Geometry check sheet. Reference: the model listing, model coordinates, mm. Face numbers are marked on the shaded views. A direction names the side the tool comes from. Give positions to 0.01 mm unless a question says otherwise; leave off trailing zeros. Loops run counter-clockwise (first coordinate to the right, second up) from the corner with the lowest first, then second, coordinate; pieces in that order, holes last.
```python
from build123d import *

# Parameters (mm, degrees)
F0_W        = 42
F0_H        = 42
F0_R        = 1.4
F0_R_2      = 11.5
F1_DEPTH    = 5
F2_T        = 2.5
F3_T1_DEPTH = 5
F4_DEPTH    = 5
F5_DEPTH    = 25


# Not quite as in the source:
# - a fillet or chamfer that OpenCascade refuses, or shapes differently, is made with other operations: its cross-section is extruded or revolved along the edge and cut away or added


with BuildPart() as f1:
    # F0 (on Top) → F1 (new body)
    with BuildSketch(Plane.XY):
        with Locations((-20.8238260887, 8.1392613277)):
            Rectangle(F0_W, F0_H)
        with Locations((-36.3238260887, -7.3607386723)):
            Circle(F0_R, mode=Mode.SUBTRACT)
        with Locations((-5.3238260887, -7.3607386723)):
            Circle(F0_R, mode=Mode.SUBTRACT)
        with Locations((-36.3238260887, 23.6392613277)):
            Circle(F0_R, mode=Mode.SUBTRACT)
        with Locations((-20.8238260887, 8.1392613277)):
            Circle(F0_R_2, mode=Mode.SUBTRACT)
        with Locations((-5.3238260887, 23.6392613277)):
            Circle(F0_R, mode=Mode.SUBTRACT)
        with Locations((-20.8238260887, 8.1392613277)):
            Circle(F0_R_2)
        with Locations((-36.3238260887, 23.6392613277)):
            Circle(F0_R)
        with Locations((-5.3238260887, 23.6392613277)):
            Circle(F0_R)
        with Locations((-5.3238260887, -7.3607386723)):
            Circle(F0_R)
        with Locations((-36.3238260887, -7.3607386723)):
            Circle(F0_R)
    extrude(amount=F1_DEPTH)

    # F2
    f2_openings = [f1.faces().sort_by_distance(p)[0] for p in [
        (-20.823826, 8.139261, 5),
    ]]
    offset(amount=F2_T, openings=f2_openings, kind=Kind.INTERSECTION)

    # F3: chamfer of 5 on 4 edges, made by hand

    # F3_s2 → F3_t1 (join)
    with BuildSketch(Plane.XY):
        Polygon((0.1761739113, -7.8607386723), (-4.8238260887, -12.8607386723), (0.1761739113, -12.8607386723), align=None)
        Polygon((0.1761739113, 24.1392613277), (-4.8238260887, 29.1392613277), (0.1761739113, 29.1392613277), align=None)
        Polygon((-36.8238260887, 29.1392613277), (-41.8238260887, 24.1392613277), (-41.8238260887, 29.1392613277), align=None)
        Polygon((-41.8238260887, -7.8607386723), (-36.8238260887, -12.8607386723), (-41.8238260887, -12.8607386723), align=None)
    extrude(amount=F3_T1_DEPTH)

    # F0 (on Top) → F4 (join)
    with BuildSketch(Plane.XY):
        with Locations((-20.8238260887, 8.1392613277)):
            Circle(F0_R_2)
    extrude(amount=F4_DEPTH)

    # F0 (on Top) → F5 (cut)
    with BuildSketch(Plane.XY):
        with Locations((-36.3238260887, -7.3607386723)):
            Circle(F0_R)
        with Locations((-36.3238260887, 23.6392613277)):
            Circle(F0_R)
        with Locations((-5.3238260887, 23.6392613277)):
            Circle(F0_R)
        with Locations((-5.3238260887, -7.3607386723)):
            Circle(F0_R)
    extrude(amount=-F5_DEPTH, mode=Mode.SUBTRACT)


solid = f1.part
```
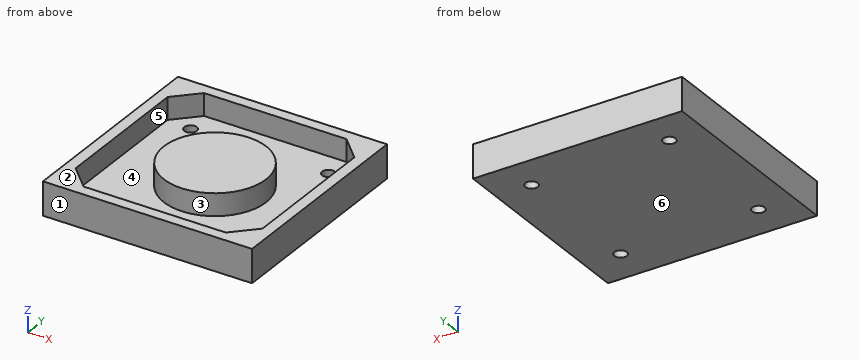
1) Sectioned sample at C-C on x = -13. Enter the section's corners in (y, z).
2) Sectioned sample at A-A on z = 1.5. Enter the section's corners in (x, y).
3) Sectioned sample at B-B on y = 7. Enter the section's corners in (x, z), plus the area to 3 significant figures.
4) Tool access check on the marked faces 5 and 6. Record the directions out of +Z, -Z, +X, -X, +Y, -Y that give a thin tool (end or side, any length) a straight path to the whole face; none if there is none.
5) Depth check by flat-ended pin: P1, Ø4.5, axis at x = -5.32, y = -7.36, coming from the -Z side; P2, Ø10, axis at x = -9.5, y = 24, coming from the +Z side. Enter the tip coordinate at first touch or a pass-through.
6) Mould release check, pull along Y, two halves, no side actions. Record for the marked faces 1, 2, 3 and 4: +Y half, -Y half, draft (parallel to the pull), parting line (faces both ways), or undercut.
7) Scan lines: line 1 along Y through (x, z) = (-21, 3.5); line 2 along Y through (x, z) = (-9, 3.75); line 3 along X through (y, z) = (-4, 0.25). Record each from-to range of solid material in increasing order.
Determined:
1. outline: (-15.36, -2.5) - (31.64, -2.5) - (31.64, 5) - (29.14, 5) - (29.14, 0) - (16.57, 0) - (16.57, 5) - (-0.29, 5) - (-0.29, 0) - (-12.86, 0) - (-12.86, 5) - (-15.36, 5) - close
2. outline: (-44.32, -15.36) - (2.68, -15.36) - (2.68, 31.64) - (-44.32, 31.64) - close; circle Ø23 at (-20.82, 8.14); hole (-41.82, -7.86) - (-36.82, -12.86) - (-4.82, -12.86) - (0.18, -7.86) - (0.18, 24.14) - (-4.82, 29.14) - (-36.82, 29.14) - (-41.82, 24.14) - close
3. outline: (-44.32, -2.5) - (2.68, -2.5) - (2.68, 5) - (0.18, 5) - (0.18, 0) - (-9.38, 0) - (-9.38, 5) - (-32.27, 5) - (-32.27, 0) - (-41.82, 0) - (-41.82, 5) - (-44.32, 5) - close
3. area: 257 mm2
4. face 5: +Z
4. face 6: -Z, +X, -X, +Y, -Y
5. P1: stops at z = -2.5
5. P2: stops at z = 0
6. face 1: -Y half
6. face 2: draft
6. face 3: undercut
6. face 4: undercut
7. line 1: y = -15.36 to -12.86, -3.36 to 19.64, 29.14 to 31.64
7. line 2: y = -15.36 to -12.86, 29.14 to 31.64
7. line 3: x = -44.32 to -41.82, 0.18 to 2.68
